Could you check a few things on this model? Use its own coordinates, in mm. Coordinates: 2 decimals unless noted, no trailing zeros. Order: outer loops, then holes, each group sorted by start corner. A loop starts at its lowest first (then second) coordinate and runs counter-clockwise, first axis right, second up. Notation, with made-up numbers: (77, -39) - (90, -39) arc R17 cw to (90, -7) - close; hole circle Ø6 at (-20, 64). An arc over 180 degrees is marked (long way). One line per item, written item: value.
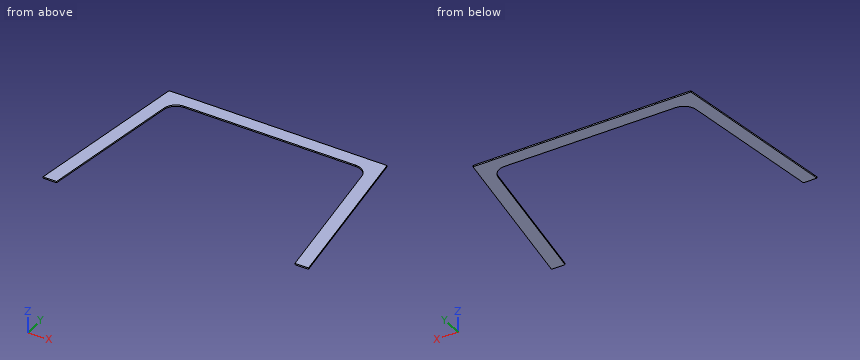
Autodesk Inventor part; units mm, degrees
ref_plane "YZ Plane" through (0, 0, 0) normal (1, 0, 0) x (0, 1, 0)
ref_plane "XZ Plane" through (0, 0, 0) normal (0, 1, 0) x (-1, 0, 0)
ref_plane "XY Plane" through (0, 0, 0) normal (0, 0, 1) x (1, 0, 0)
sketch "Sketch1" plane through (0, 0, 0) normal (0, 0, 1) x (1, 0, 0)
  line L0 (0, 60) -> (0, -80) construction
  line L1 (-110.88, 0) -> (110.88, 0) construction
  line L2 (-79.2, -60) -> (79.2, -60)
  line L3 (79.2, -60) -> (65, 40)
  line L4 (-65, 40) -> (65, 40)
  line L5 (-65, 40) -> (-79.2, -60)
  point P0 (0, 0)
  dimension "d0" = 158.4
  dimension "d9" = 130
  dimension "d10" = 60
  dimension "d11" = 100
extrude "Extrusion1" add sketch "Sketch1" along normal mid plane 0.8
sketch "Esquisse2" plane through (0, 0, 0.4) normal (0, 0, 1) x (1, 0, 0)
  line L0 (-79.2, -60) -> (79.2, -60) construction
  line L1 (79.2, -60) -> (65, 40) construction
  line L2 (65, 40) -> (-65, 40) construction
  line L3 (-65, 40) -> (-79.2, -60) construction
  line L4 (0, 60) -> (0, -80) construction
  line L5 (-110.88, 0) -> (110.88, 0) construction
  line L6 (-51.1115, 32) -> (51.1115, 32)
  line L7 (-59.032, 25.1247) -> (-71.1197, -60)
  line L8 (59.032, 25.1247) -> (71.1197, -60)
  arc A0 (-51.1115, 32) -> (-59.032, 25.1247) centre (-51.1115, 24) ccw
  arc A1 (59.032, 25.1247) -> (51.1115, 32) centre (51.1115, 24) ccw
  line L9 (-71.1197, -60) -> (71.1197, -60)
  point P0 (0, 0)
  dimension "d12" = 8
  dimension "d15" = 8
  dimension "d16" = 8
extrude "Extrusion2" cut sketch "Esquisse2" against normal through all
properties part number "Cabine_Vitre_Avant_Haut" material "PVC-U"
Item 1: I want a section at A-A on y = -48.5. Please give me the cut outline in (x, z), then the cut area to 3 significant figures.
Conclusion:
outline: (-77.57, -0.4) - (-69.49, -0.4) - (-69.49, 0.4) - (-77.57, 0.4) - close; (69.49, -0.4) - (77.57, -0.4) - (77.57, 0.4) - (69.49, 0.4) - close
area: 12.9 mm²
Item 2: I want a section at B-B on z = -0.25. Please give me the cut outline in (x, y), then the cut area to 3 significant figures.
Conclusion:
outline: (-79.2, -60) - (-71.12, -60) - (-59.03, 25.12) arc R8 cw to (-51.11, 32) - (51.11, 32) arc R8 cw to (59.03, 25.12) - (71.12, -60) - (79.2, -60) - (65, 40) - (-65, 40) - close
area: 2,560 mm²
Item 3: I want a section at C-C on x = -5. Please give me the cut outline in (y, z), then the cut area to 3 significant figures.
Conclusion:
outline: (32, -0.4) - (40, -0.4) - (40, 0.4) - (32, 0.4) - close
area: 6.40 mm²
Item 4: If I drill on probe 1 along Y at (x, z) = (-22, 0.15); probe 2 along X at (y, z) = (24, -0.2); probe 3 along X at (y, z) = (2.5, -0.25) (3 decimals), over which ranges is the centre line in solid material (lowest first)?
Conclusion:
probe 1: 32 to 40
probe 2: -67.27 to -59.19, 59.19 to 67.27
probe 3: -70.325 to -62.245, 62.245 to 70.325
Item 5: I want a section at D-D on x = -69. Please give me the cut outline in (y, z).
Conclusion:
outline: (-45.07, -0.4) - (11.83, -0.4) - (11.83, 0.4) - (-45.07, 0.4) - close
